Design review of the part built by this model. Coordinates are the model's own, in mm. A direction names the side the tool comes from. Round coordinates to 2 decimals unless told otherwise and drop trailing zeros. Loops run counter-clockwise (first coordinate to the right, second up) from the corner with the lowest first, then second, coordinate; pieces in that order, holes last. Notation, with made-up numbers: (16.25, 58) - (73.25, 58) arc R23 cw to (73.25, 87) - close; hole circle Ø3 at (0.5, 85.5). An arc over 180 degrees is marked (long way). Return JSON: item names as keys, results as strings. Group by question number.
(1) We need section B-B, the plane z = 24.5. Write out the cut boundary in (x, y).
(2) We need section C-C, the plane y = 3.5. Write out the cut boundary in (x, z), and give its area (3 significant figures).
(3) We need section A-A, the plane x = 47. Write out the cut boundary in (y, z), and give its area (3 significant figures).
(4) For faces 1 (the cylindrical face through (1.91, 1.81, 3.13)), 2 (the flat face through (28, 9, 6.35)), list the 3-axis set-ups (+Z, -Z, +X, -X, +Y, -Y) from which the entire face can be reached by the end or side of a thin tool; tool diameter is ignored.
(5) Wall thickness on L1, parallel to Y at x = 49, z = 63; L2, parallel to Z at x = 15.5, y = 10.5: over which ranges is each line inside the solid? List them lowest first. Write a range as [from, to].
(6) Clearance check with flat-ended pins moving along their axes: pin 1 (2 mm diameter, centred on y = 18, z = 25.5, fed in from +X); pin 2 (5 mm diameter, centred on x = 48, y = 4.5, fed in from +Z); pin 3 (10 mm diameter, centred on x = 27, z = 28, fed in from -Y); pin 4 (8 mm diameter, centred on x = 14, y = 37, fed in from -Z). State where each tip first meets the part, or that it passes through.
from build123d import *

# Parameters (mm, degrees)
F0_W     = 69.85
F0_H     = 69.85
F1_DEPTH = 44.45
F2_W     = 69.85
F2_H     = 63.5
F3_DEPTH = 19.05
F5_DEPTH = 69.85
F7_DEPTH = 25.4


with BuildPart() as f1:
    # F0 (on Front) → F1 (new body)
    with BuildSketch(Plane.XZ):
        with Locations((34.925, 34.925)):
            Rectangle(F0_W, F0_H)
    extrude(amount=-F1_DEPTH)

    # F2 (on face) → F3 (cut)
    with BuildSketch(Plane.XZ):
        with Locations((34.925, 38.1)):
            Rectangle(F2_W, F2_H)
    extrude(amount=-F3_DEPTH, mode=Mode.SUBTRACT)

    # F4 (on Top) → F5 (cut)
    with BuildSketch(Plane.XY):
        with BuildLine():
            ThreePointArc((57.15, 7.143745), (54.338231, 2.119989), (48.985679, 0))
            Line((48.985679, 0), (69.85, 0))
            Line((69.85, 0), (69.85, 44.45))
            Line((69.85, 44.45), (57.15, 44.45))
            Line((57.15, 44.45), (57.15, 7.143745))
        make_face()
    extrude(amount=F5_DEPTH, mode=Mode.SUBTRACT)

    # F6 (on Top) → F7 (cut)
    with BuildSketch(Plane.XY):
        with BuildLine():
            ThreePointArc((6.35, 0), (1.859872, 1.859872), (0, 6.35))
            Line((0, 6.35), (0, 0))
            Line((0, 0), (6.35, 0))
        make_face()
    extrude(amount=F7_DEPTH, mode=Mode.SUBTRACT)


solid = f1.part
Solutions:
{
 "1": {"outline": "(0, 19.05) - (57.15, 19.05) - (57.15, 44.45) - (0, 44.45) - close"},
 "2": {"outline": "(0.68, 0) - (55.61, 0) - (55.61, 6.35) - (0.68, 6.35) - close", "area": "349 mm^2"},
 "3": {"outline": "(0, 0) - (44.45, 0) - (44.45, 69.85) - (19.05, 69.85) - (19.05, 6.35) - (0, 6.35) - close", "area": "1,900 mm^2"},
 "4": {"face 1": "+Z, -Z, -X, -Y", "face 2": "+Z, +X, -X, -Y"},
 "5": {"L1": "[19.05, 44.45]", "L2": "[0, 6.35]"},
 "6": {"pin 1": "through", "pin 2": "z = 6.35", "pin 3": "y = 19.05", "pin 4": "z = 0"}
}
